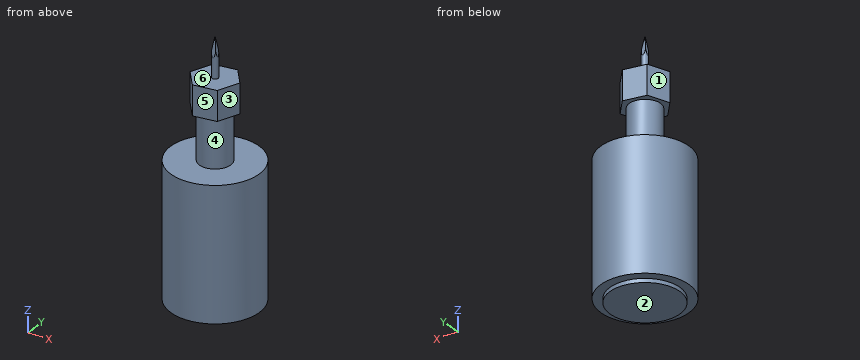
from build123d import *

# Parameters (mm, degrees)
SKETCH1_R                      = 22.5
BOSS_EXTRUDE1_DEPTH            = 67
SKETCH2_R                      = 8
BOSS_EXTRUDE2_DEPTH            = 40
BOSS_EXTRUDE3_DEPTH            = 15
SKETCH4_R                      = 1.5875
BOSS_EXTRUDE4_DEPTH            = 20
CUT_EXTRUDE1_REACH             = 24.5
CUT_EXTRUDE1_DIRECTION_2_REACH = 24.5
CUT_EXTRUDE2_REACH             = 24.5
CUT_EXTRUDE2_DIRECTION_2_REACH = 24.5
SKETCH7_R                      = 17.895926968
BOSS_EXTRUDE5_DEPTH            = 2


with BuildPart() as part:
    # Sketch1 → Boss-Extrude1 (new body)
    with BuildSketch(Plane.XY):
        Circle(SKETCH1_R)
    extrude(amount=BOSS_EXTRUDE1_DEPTH)

    # Sketch2 → Boss-Extrude2 (add)
    with BuildSketch(Plane.XY.offset(67)):
        Circle(SKETCH2_R)
    extrude(amount=BOSS_EXTRUDE2_DEPTH)

    # Sketch3 → Boss-Extrude3 (add)
    with BuildSketch(Plane.XY.offset(107)):
        Polygon((11.534146379, 1.930154149), (4.095510664, 10.95394085), (-7.438635716, 9.023786701), (-11.534146379, -1.930154149), (-4.095510664, -10.95394085), (7.438635716, -9.023786701), align=None)
    extrude(amount=-BOSS_EXTRUDE3_DEPTH)

    # Sketch4 → Boss-Extrude4 (add)
    with BuildSketch(Plane.XY.offset(107)):
        Circle(SKETCH4_R)
    extrude(amount=BOSS_EXTRUDE4_DEPTH)

    # Sketch5 → Cut-Extrude1 (cut, up to next)
    with BuildSketch(Plane(origin=(0, 0, 0), x_dir=(1, 0, 0), z_dir=(0, 1, 0)), mode=Mode.PRIVATE) as cut_extrude1_sk1:
        Polygon((-1.5875, -127), (0, -127), (-1.5875, -117), align=None)
    cut_extrude1_tool1 = extrude(cut_extrude1_sk1.sketch, amount=-CUT_EXTRUDE1_REACH, mode=Mode.PRIVATE) & part.part
    add(cut_extrude1_tool1.solids().sort_by_distance((-1.058333, 0, 123.666667))[0], mode=Mode.SUBTRACT)
    # Sketch5 → Cut-Extrude1 (cut, up to next)
    with BuildSketch(Plane(origin=(0, 0, 0), x_dir=(1, 0, 0), z_dir=(0, 1, 0)), mode=Mode.PRIVATE) as cut_extrude1_sk2:
        Polygon((1.630697713, -117), (0, -127), (1.5875, -127), align=None)
    cut_extrude1_tool2 = extrude(cut_extrude1_sk2.sketch, amount=-CUT_EXTRUDE1_REACH, mode=Mode.PRIVATE) & part.part
    add(cut_extrude1_tool2.solids().sort_by_distance((1.072733, 0, 123.666667))[0], mode=Mode.SUBTRACT)

    # Sketch5 → Cut-Extrude1 direction 2 (cut, up to next)
    with BuildSketch(Plane(origin=(0, 0, 0), x_dir=(1, 0, 0), z_dir=(0, 1, 0)), mode=Mode.PRIVATE) as cut_extrude1_direction_2_sk1:
        Polygon((-1.5875, -127), (0, -127), (-1.5875, -117), align=None)
    cut_extrude1_direction_2_tool1 = extrude(cut_extrude1_direction_2_sk1.sketch, amount=CUT_EXTRUDE1_DIRECTION_2_REACH, mode=Mode.PRIVATE) & part.part
    add(cut_extrude1_direction_2_tool1.solids().sort_by_distance((-1.058333, 0, 123.666667))[0], mode=Mode.SUBTRACT)
    # Sketch5 → Cut-Extrude1 direction 2 (cut, up to next)
    with BuildSketch(Plane(origin=(0, 0, 0), x_dir=(1, 0, 0), z_dir=(0, 1, 0)), mode=Mode.PRIVATE) as cut_extrude1_direction_2_sk2:
        Polygon((1.630697713, -117), (0, -127), (1.5875, -127), align=None)
    cut_extrude1_direction_2_tool2 = extrude(cut_extrude1_direction_2_sk2.sketch, amount=CUT_EXTRUDE1_DIRECTION_2_REACH, mode=Mode.PRIVATE) & part.part
    add(cut_extrude1_direction_2_tool2.solids().sort_by_distance((1.072733, 0, 123.666667))[0], mode=Mode.SUBTRACT)

    # Sketch6 → Cut-Extrude2 (cut, up to next)
    with BuildSketch(Plane(origin=(0, 0, 0), x_dir=(0, 0, -1), z_dir=(1, 0, 0)), mode=Mode.PRIVATE) as cut_extrude2_sk1:
        Polygon((-127, -1.5875), (-117, -1.5875), (-127, 0), align=None)
    cut_extrude2_tool1 = extrude(cut_extrude2_sk1.sketch, amount=-CUT_EXTRUDE2_REACH, mode=Mode.PRIVATE) & part.part
    add(cut_extrude2_tool1.solids().sort_by_distance((0, -1.058333, 123.666667))[0], mode=Mode.SUBTRACT)
    # Sketch6 → Cut-Extrude2 (cut, up to next)
    with BuildSketch(Plane(origin=(0, 0, 0), x_dir=(0, 0, -1), z_dir=(1, 0, 0)), mode=Mode.PRIVATE) as cut_extrude2_sk2:
        Polygon((-127, 0), (-117, 1.5875), (-127, 1.5875), align=None)
    cut_extrude2_tool2 = extrude(cut_extrude2_sk2.sketch, amount=-CUT_EXTRUDE2_REACH, mode=Mode.PRIVATE) & part.part
    add(cut_extrude2_tool2.solids().sort_by_distance((0, 1.058333, 123.666667))[0], mode=Mode.SUBTRACT)

    # Sketch6 → Cut-Extrude2 direction 2 (cut, up to next)
    with BuildSketch(Plane(origin=(0, 0, 0), x_dir=(0, 0, -1), z_dir=(1, 0, 0)), mode=Mode.PRIVATE) as cut_extrude2_direction_2_sk1:
        Polygon((-127, -1.5875), (-117, -1.5875), (-127, 0), align=None)
    cut_extrude2_direction_2_tool1 = extrude(cut_extrude2_direction_2_sk1.sketch, amount=CUT_EXTRUDE2_DIRECTION_2_REACH, mode=Mode.PRIVATE) & part.part
    add(cut_extrude2_direction_2_tool1.solids().sort_by_distance((0, -1.058333, 123.666667))[0], mode=Mode.SUBTRACT)
    # Sketch6 → Cut-Extrude2 direction 2 (cut, up to next)
    with BuildSketch(Plane(origin=(0, 0, 0), x_dir=(0, 0, -1), z_dir=(1, 0, 0)), mode=Mode.PRIVATE) as cut_extrude2_direction_2_sk2:
        Polygon((-127, 0), (-117, 1.5875), (-127, 1.5875), align=None)
    cut_extrude2_direction_2_tool2 = extrude(cut_extrude2_direction_2_sk2.sketch, amount=CUT_EXTRUDE2_DIRECTION_2_REACH, mode=Mode.PRIVATE) & part.part
    add(cut_extrude2_direction_2_tool2.solids().sort_by_distance((0, 1.058333, 123.666667))[0], mode=Mode.SUBTRACT)

    # Sketch7 → Boss-Extrude5 (add)
    with BuildSketch(Plane(origin=(0, 0, 0), x_dir=(-1, 0, 0), z_dir=(0, 0, -1))):
        Circle(SKETCH7_R)
    extrude(amount=BOSS_EXTRUDE5_DEPTH)


solid = part.part
The model under review builds one solid part; all positions refer to its coordinate system, in mm. Face numbers are marked on the shaded views. A direction names the side the tool comes from. Round coordinates to 2 decimals unless told otherwise and drop trailing zeros. Write each loop counter-clockwise with the first axis right and the second up, starting at its lowest first coordinate (ties: lowest second). Pieces come first, ordered by that corner, then holes. Notation, with made-up numbers: M 23.25,80.5 L 37.25,80.5 A33 cw 37.25,109.5 Z; hole C 34,41 d5. An arc over 180 degrees is marked long. Use a Markdown table: item, result. Add a question column.
Q1. To check wall thickness, follow line 1 (Z direction, x = 8.5, y = -6); line 2 (Z direction, x = 2.5, y = -7); line 3 (Z direction, x = -13, y = -7). State the ranges of each line that lie inside material, in increasing order.
Q2. We need section D-D, the plane z = 81. State the section outline as (x, y) points.
Q3. The part is to be moulded in two halves that separate along Z. For the marked faces 4, 5 and 6, say which applies: pulls with the +Z half, pulls with the -Z half, needs draft (parallel to the pull), parting line crosses it, or undercut.
Q4. Insertion check: pin 1 (10 mm diameter, centred on x = -15, z = 32.5, fed in from -Y); pin 2 (5 mm diameter, centred on y = -10.5, z = 52.5, fed in from -X); pin 3 (11 mm diameter, centred on x = -2, y = -2, fed in from +Z); pin 4 (12 mm diameter, centred on y = -14, z = 35.5, fed in from +X). Each pin has a flat end and moves straight along its axis. Give the tip position at first contact, or say it passes through.
Q5. Machinability: for the marked faces 1, 2 and 3, which of the approach directions +Z, -Z, +X, -X, +Y, -Y give a long, thin tool a straight path to every point of the face, cutting with its end or side? Answer none if there is none.
Q6. We need section C-C, the plane z = 30. State the section outline as (x, y) points, plus the area to 3 significant figures.
Q7. We need section A-A, the plane y = -15. State the section outline as (x, z) points.
Findings below:
| question | item | result |
|---|---|---|
| 1 | line 1 | z = -2 to 67, 92 to 107 |
| 1 | line 2 | z = -2 to 107 |
| 1 | line 3 | z = -2 to 67 |
| 2 | outline | C 0,0 d16 |
| 3 | face 4 | undercut |
| 3 | face 5 | needs draft |
| 3 | face 6 | pulls with the +Z half |
| 4 | pin 1 | stops at y = -20.16 |
| 4 | pin 2 | stops at x = -21.03 |
| 4 | pin 3 | stops at z = 127 |
| 4 | pin 4 | stops at x = 21.03 |
| 5 | face 1 | +Z, -X, +Y |
| 5 | face 2 | -Z, +X, -X, +Y, -Y |
| 5 | face 3 | +Z, +X, -Y |
| 6 | outline | C 0,0 d45 |
| 6 | area | 1,590 mm² |
| 7 | outline | M -16.77,0 L -9.76,0 L -9.76,-2 L 9.76,-2 L 9.76,0 L 16.77,0 L 16.77,67 L -16.77,67 Z |
